from build123d import *

# Parameters (mm, degrees)
PAD001_START         = 10
PAD001_DEPTH         = 15
POCKET004_DEPTH      = 7.501
POCKET004_DEPTH_BACK = 7.501
PAD002_DEPTH         = 15
POCKET005_DEPTH      = 2.15
SKETCH011_R          = 1.7
HOLE001_DEPTH        = 12.7504949366
SKETCH012_R          = 1.9
PAD003_DEPTH         = 4.5
CHAMFER_SIZE         = 0.5
FILLET001_R          = 1


with BuildPart() as part:
    # Sketch007 → Pad001 (new body)
    with BuildSketch(Plane.XY.offset(PAD001_START)):
        Polygon((-7, -6), (-1, -6), (-1, -7.5), (4, -7.5), (4, -6), (7, -6), (7, -1), (4, -1), (4, 7.5), (-1, 7.5), (-1, -1), (-7, -1), align=None)
    extrude(amount=PAD001_DEPTH)

    # Sketch008 → Pocket004 (cut, two sides)
    with BuildSketch(Plane.XZ) as pocket004_sk:
        Polygon((-7, 25), (7, 11), (7, 25), align=None)
    extrude(amount=-POCKET004_DEPTH, mode=Mode.SUBTRACT)
    extrude(pocket004_sk.sketch, amount=POCKET004_DEPTH_BACK, mode=Mode.SUBTRACT)

    # Sketch009 (on Face8 of Pocket004) → Pad002 (join)
    with BuildSketch(Plane.XZ.offset(7.5)):
        Polygon((-7, 25), (7, 11), (7, 18.0710678119), (-7, 32.0710678119), align=None)
    extrude(amount=-PAD002_DEPTH)

    # Sketch010 (on Face12 of Pad002) → Pocket005 (cut)
    with BuildSketch(Plane(origin=(9, 0, 9), x_dir=(0.7071067812, 0, -0.7071067812), z_dir=(-0.7071067812, 0, -0.7071067812))):
        Polygon((-21.5619467058, -2.3333103769), (-20.6952570827, -5.5678400847), (-17.4607273749, -6.4345297078), (-15.0928872902, -4.0666896231), (-15.9595769133, -0.8321599153), (-19.1941066211, 0.0345297078), align=None)
    extrude(amount=-POCKET005_DEPTH, mode=Mode.SUBTRACT)

    # Sketch011 (on Face29 of Pocket005) → Hole001 (cut, through all)
    with BuildSketch(Plane(origin=(10.5202795796, 0, 10.5202795796), x_dir=(0, -1, 0), z_dir=(-0.7071067812, 0, -0.7071067812))):
        with Locations((-3.2, 18.327416998)):
            Circle(SKETCH011_R)
    extrude(amount=-HOLE001_DEPTH, mode=Mode.SUBTRACT)

    # Sketch012 (on Face9 of Hole001) → Pad003 (join)
    with BuildSketch(Plane(origin=(12.5355339059, 0, 12.5355339059), x_dir=(0.7071067812, 0, -0.7071067812), z_dir=(0.7071067812, 0, 0.7071067812))):
        with Locations((-22.027416998, -3.8)):
            Circle(SKETCH012_R)
        with Locations((-11.127416998, -0.3)):
            Circle(SKETCH012_R)
    extrude(amount=PAD003_DEPTH)

    # Chamfer
    chamfer_edges = [part.edges().sort_by_distance(p)[0] for p in [
        (-1.201724, -3.8, 32.636753),
        (6.50574, -0.3, 24.929289),
    ]]
    chamfer(chamfer_edges, length=CHAMFER_SIZE)

    # Fillet001
    fillet001_edges = [part.edges().sort_by_distance(p)[0] for p in [
        (-7, 0, 32.071068),
        (7, 3.25, 11),
        (7, -6.75, 11),
    ]]
    fillet(fillet001_edges, radius=FILLET001_R)


with BuildPart() as part_1:
    # Body001 placement: moved
    add(part.part.moved(Location((0, 0, -3))))


solid = part_1.part
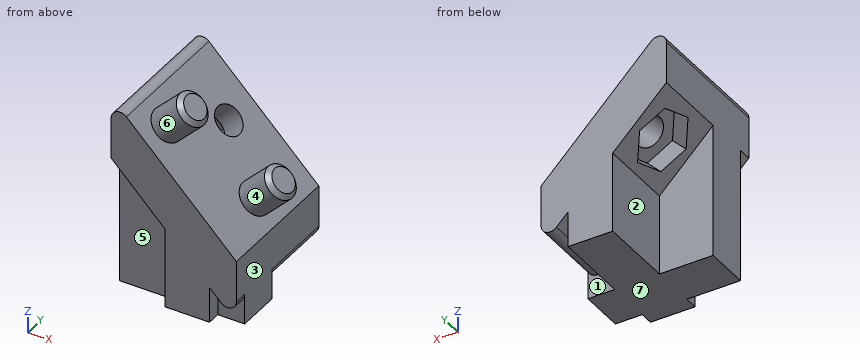
Geometry check sheet. Reference: the model listing, model coordinates, mm. Face numbers are marked on the shaded views. A direction names the side the tool comes from. Give positions to 0.01 mm unless a question says otherwise; leave off trailing zeros. Write each loop counter-clockwise with the first axis right and the second up, starting at its lowest first coordinate (ties: lowest second). Pieces come first, ordered by that corner, then holes. Notation, with made-up numbers: M 75,35.5 L 127,35.5 A19 cw 127,48.5 Z; hole C 43,17 d3. An arc over 180 degrees is marked long. Answer as CSV lines item,"result". Start each with the question number.
Q1. Section check C-C, the plane z = 15.5. Record the cut outline in (x, y), then the cut area to 3 significant figures.
Q2. Release check for a two-part mould opening along Z. For the marked faces 4, 5, 6 and 7 record: pulls with the +Z half, pulls with the -Z half, needs draft (parallel to the pull), parting line crosses it, or undercut.
Q3. Section check B-B, the plane z = 11.25. Record the cut outline in (x, y), then the cut area to 3 significant figures.
Q4. Tool access check on the marked faces 1, 2 and 3. Record the directions out of +Z, -Z, +X, -X, +Y, -Y that give a thin tool (end or side, any length) a straight path to the whole face; none if there is none.
Q5. Material ranges on L1, parallel to X at y = -3.25, z = 13; L2, parallel to Y at x = -2.5, z = 14.5; L3, parallel to X at y = 6.25, z = 9.75, recorded low to high.
Q6. Section check D-D, the plane x = 1.75. Record the cut outline in (y, z).
Q7. Go/stop test with flat-tipped pins: pin 1 (0.9 mm diameter, centred on x = 5, z = 8.5, fed in from -Y); pin 2 (1.2 mm diameter, centred on y = 3.5, z = 10, fed in from +X); pin 3 (2 mm diameter, centred on x = 5, z = 17.5, fed in from +Y); pin 4 (1.5 mm diameter, centred on x = 6, z = 8.5, fed in from +Y). Record where each tip stops, or that it passes through.
Q8. Section check A-A, the plane y = 3.75. Record the cut outline in (x, z), then the cut area to 3 significant figures.
Geometry says:
1,outline,"M -7,-6 L -1,-6 L -1,-7.5 L 6.57,-7.5 L 6.57,7.5 L -1,7.5 L -1,-1 L -7,-1 Z"
1,area,"144 mm^2"
2,face 4,"undercut"
2,face 5,"needs draft"
2,face 6,"undercut"
2,face 7,"pulls with the -Z half"
3,outline,"M -7,-6 L -1,-6 L -1,-7.5 L 7,-7.5 L 7,7.5 L -1,7.5 L -1,-1 L -7,-1 Z"
3,area,"150 mm^2"
4,face 1,"-Z, +Y"
4,face 2,"-Z, -X, +Y"
4,face 3,"-Z, +X, +Y, -Y"
5,L1,"-7 to 7"
5,L2,"-6 to -1"
5,L3,"-1 to 4, 5.25 to 6.75"
6,outline,"M -7.5,7 L 7.5,7 L 7.5,20.32 L -7.5,20.32 Z"
7,pin 1,"y = -6"
7,pin 2,"x = 7"
7,pin 3,"y = 7.5"
7,pin 4,"y = -1"
8,outline,"M -7,22 L -5.98,20.98 L -4.46,22.5 L -3.58,21.62 L -1.56,23.63 L -5.29,27.36 A1 ccw -7,26.66 Z; M -1.73,16.73 L -1,16 L -1,7 L 4,7 L 4,11 L 5.29,9.71 A1 ccw 7,10.41 L 7,15.07 L 0.71,21.36 L -1.3,19.34 L -0.21,18.25 Z"
8,area,"107 mm^2"
